```python
from build123d import *

# Parameters (mm, degrees)
SKETCH12_W          = 26
SKETCH12_H          = 26
BOSS_EXTRUDE7_DEPTH = 3
SKETCH12_6_W        = 32
SKETCH12_6_H        = 32
SKETCH12_6_W_2      = 26
SKETCH12_6_H_2      = 26
BOSS_EXTRUDE8_DEPTH = 12
SKETCH12_7_W        = 3.9
SKETCH12_7_H        = 3.9
CUT_EXTRUDE34_DEPTH = 3
SKETCH12_8_W        = 4.3
SKETCH12_8_H        = 4.3
CUT_EXTRUDE36_DEPTH = 1.5
SKETCH23_R          = 2
CUT_EXTRUDE47_DEPTH = 32
SKETCH24_W          = 3.4
SKETCH24_H          = 3.4
CUT_EXTRUDE48_DEPTH = 3
SKETCH24_3_W        = 3.8
SKETCH24_3_H        = 3.8
CUT_EXTRUDE49_DEPTH = 1.5
SKETCH25_R          = 1.25
CUT_EXTRUDE50_DEPTH = 3


with BuildPart() as part:
    # Sketch12 → Boss-Extrude7 (new body)
    with BuildSketch(Plane(origin=(0, 0, 0), x_dir=(1, 0, 0), z_dir=(0, 1, 0))):
        Rectangle(SKETCH12_W, SKETCH12_H)
    extrude(amount=BOSS_EXTRUDE7_DEPTH)

    # Sketch12<6> → Boss-Extrude8 (add)
    with BuildSketch(Plane(origin=(0, 0, 0), x_dir=(1, 0, 0), z_dir=(0, 1, 0))):
        Rectangle(SKETCH12_6_W, SKETCH12_6_H)
        Rectangle(SKETCH12_6_W_2, SKETCH12_6_H_2, mode=Mode.SUBTRACT)
    extrude(amount=BOSS_EXTRUDE8_DEPTH)

    # Sketch12<7> → Cut-Extrude34 (cut)
    with BuildSketch(Plane(origin=(0, 0, 0), x_dir=(1, 0, 0), z_dir=(0, 1, 0))):
        Rectangle(SKETCH12_7_W, SKETCH12_7_H)
    extrude(amount=CUT_EXTRUDE34_DEPTH, mode=Mode.SUBTRACT)

    # Sketch12<8> → Cut-Extrude36 (cut)
    with BuildSketch(Plane(origin=(0, 0, 0), x_dir=(1, 0, 0), z_dir=(0, 1, 0))):
        Rectangle(SKETCH12_8_W, SKETCH12_8_H)
    extrude(amount=CUT_EXTRUDE36_DEPTH, mode=Mode.SUBTRACT)

    # Sketch23 → Cut-Extrude47 (cut)
    with BuildSketch(Plane(origin=(16, 0, 0), x_dir=(0, 0, -1), z_dir=(1, 0, 0))):
        with Locations((0, 9)):
            Circle(SKETCH23_R)
    extrude(amount=-CUT_EXTRUDE47_DEPTH, mode=Mode.SUBTRACT)

    # Sketch24 → Cut-Extrude48 (cut)
    with BuildSketch(Plane(origin=(0, 0, -16), x_dir=(-1, 0, 0), z_dir=(0, 0, -1))):
        with Locations((0, 9)):
            Rectangle(SKETCH24_W, SKETCH24_H)
    extrude(amount=-CUT_EXTRUDE48_DEPTH, mode=Mode.SUBTRACT)

    # Sketch24<3> → Cut-Extrude49 (cut)
    with BuildSketch(Plane(origin=(0, 0, -16), x_dir=(-1, 0, 0), z_dir=(0, 0, -1))):
        with Locations((0, 9)):
            Rectangle(SKETCH24_3_W, SKETCH24_3_H)
    extrude(amount=-CUT_EXTRUDE49_DEPTH, mode=Mode.SUBTRACT)

    # Sketch25 → Cut-Extrude50 (cut)
    with BuildSketch(Plane.XY.offset(16)):
        with Locations((0, 9)):
            Circle(SKETCH25_R)
    extrude(amount=-CUT_EXTRUDE50_DEPTH, mode=Mode.SUBTRACT)


solid = part.part
```
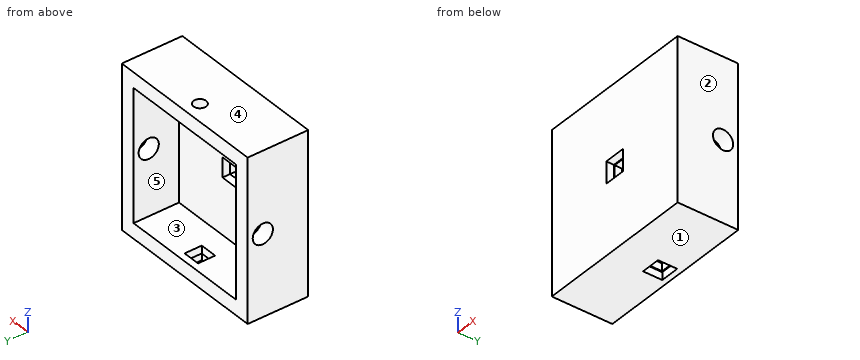
Here's how the part is built. I have some questions about the finished solid (model axes, mm). Face numbers are marked on the shaded views. A direction names the side the tool comes from. Round coordinates to 2 decimals unless told otherwise and drop trailing zeros. Order: outer loops, then holes, each group sorted by start corner. A loop starts at its lowest first (then second) coordinate and runs counter-clockwise, first axis right, second up. Notation, with made-up numbers: M -35.75,54 L -23.75,54 A17 cw -23.75,59 Z; hole C -6.5,6 d3. An arc over 180 degrees is marked long. Answer in a Markdown table with one row per item.
Item 1: Thinking about a two-plate mould opening in Z: for the marked faces 1, 2 and 3, which applies, +Z half, -Z half, draft (parallel to the pull), parting line (faces both ways), or undercut?
A:
| item | result |
|---|---|
| face 1 | -Z half |
| face 2 | draft |
| face 3 | undercut |
Item 2: I'm going to push flat-ended pins straight in: pin 1 (4.5 mm diameter, centred on x = -1, z = 0.5, fed in from -Y); pin 2 (4 mm diameter, centred on x = -8, z = -8.5, fed in from +Y). Where does each tip first touch, or does it pass through?
A:
| item | result |
|---|---|
| pin 1 | stops at y = 0 |
| pin 2 | stops at y = 3 |
Item 3: Imagine slicing it at D-D, the plane z = 0. Write out the boundary of the cut face in (x, y).
A:
| item | result |
|---|---|
| outline | M -16,0 L -2.15,0 L -2.15,1.5 L -1.95,1.5 L -1.95,3 L -13,3 L -13,7 L -16,7 Z; M -16,11 L -13,11 L -13,12 L -16,12 Z; M 1.95,1.5 L 2.15,1.5 L 2.15,0 L 16,0 L 16,7 L 13,7 L 13,3 L 1.95,3 Z; M 13,11 L 16,11 L 16,12 L 13,12 Z |
Item 4: Imagine slicing it at B-B, the plane x = 0. Write out the boundary of the cut face in (y, z).
A:
| item | result |
|---|---|
| outline | M 0,-16 L 7.1,-16 L 7.1,-14.5 L 7.3,-14.5 L 7.3,-13 L 3,-13 L 3,-1.95 L 1.5,-1.95 L 1.5,-2.15 L 0,-2.15 Z; M 0,2.15 L 1.5,2.15 L 1.5,1.95 L 3,1.95 L 3,13 L 7.75,13 L 7.75,16 L 0,16 Z; M 10.25,13 L 12,13 L 12,16 L 10.25,16 Z; M 10.7,-14.5 L 10.9,-14.5 L 10.9,-16 L 12,-16 L 12,-13 L 10.7,-13 Z |
Item 5: Imagine slicing it at A-A, the plane y = 9. Write out the boundary of the cut face in (x, z), and give its area (3 significant figures).
A:
| item | result |
|---|---|
| outline | M -16,-16 L -1.9,-16 L -1.9,-14.5 L -1.7,-14.5 L -1.7,-13 L -13,-13 L -13,-2 L -16,-2 Z; M -16,2 L -13,2 L -13,13 L -1.25,13 L -1.25,16 L -16,16 Z; M 1.25,13 L 13,13 L 13,2 L 16,2 L 16,16 L 1.25,16 Z; M 1.7,-14.5 L 1.9,-14.5 L 1.9,-16 L 16,-16 L 16,-2 L 13,-2 L 13,-13 L 1.7,-13 Z |
| area | 306 mm2 |
Item 6: If I drill on L1, parallel to Z at x = 12.5, y = 10.25; L2, parallel to Y at x = 0, z = 15, over which ranges is the centre line in solid material (lowest first)? Write a range as from..to.
A:
| item | result |
|---|---|
| L1 | z = -16..-13, 13..16 |
| L2 | y = 0..7.75, 10.25..12 |
Item 7: Imagine slicing it at C-C, the plane y = 5.5. Write out the boundary of the cut face in (x, z), and give its area (3 significant figures).
A:
| item | result |
|---|---|
| outline | M -16,-16 L 16,-16 L 16,16 L -16,16 Z; hole M -13,-13 L 13,-13 L 13,13 L -13,13 Z |
| area | 348 mm2 |
Item 8: For the marked faces 4 and 5, which set-ups out of +Z, -Z, +X, -X, +Y, -Y let a thin tool reach every point of the face, with its end or its side?
A:
| item | result |
|---|---|
| face 4 | +Z, +X, -X, +Y, -Y |
| face 5 | +Y |
